Build history of the part. All positions in model axes, mm. Face numbers are marked on the shaded views. A direction names the side the tool comes from. Round coordinates to 2 decimals unless told otherwise and drop trailing zeros. Loops run counter-clockwise (first coordinate to the right, second up) from the corner with the lowest first, then second, coordinate; pieces in that order, holes last. Notation, with made-up numbers: (62.25, 37.25) - (104.25, 37.25) arc R17 cw to (104.25, 52.25) - close; hole circle Ø8 at (27, 53). An arc over 180 degrees is marked (long way). Put each result on its own line as item: value. Start each with the question number.
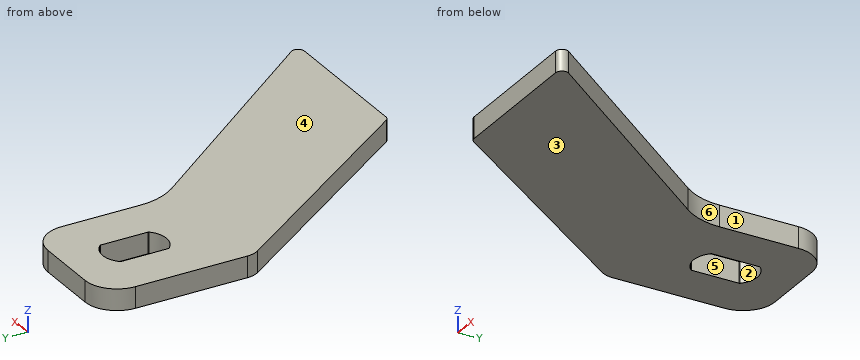
from build123d import *

# Parameters (mm, degrees)
EXTRUDE1_DEPTH = 10


with BuildPart() as part:
    # Sketch1 → Extrude1 (new body)
    with BuildSketch(Plane.XY):
        with BuildLine():
            Line((15, 32), (-15, 32))
            ThreePointArc((-15, 32), (-25.606601718, 27.606601718), (-30, 17))
            Line((-30, 17), (-30, -35.847012111))
            ThreePointArc((-30, -35.847012111), (-29.537169507, -38.854070106), (-28.191520443, -41.582776475))
            Line((-28.191520443, -41.582776475), (43.326244069, -143.720729309))
            ThreePointArc((43.326244069, -143.720729309), (44.398454362, -144.6610325), (45.783700202, -145))
            Line((45.783700202, -145), (111.775541918, -145))
            ThreePointArc((111.775541918, -145), (114.466160142, -143.326866071), (114.155601938, -140.173715713))
            Line((114.155601938, -140.173715713), (36.199399791, -38.579215104))
            ThreePointArc((36.199399791, -38.579215104), (31.592096115, -29.959556193), (30, -20.316372234))
            Line((30, -20.316372234), (30, 17))
            ThreePointArc((30, 17), (25.606601718, 27.606601718), (15, 32))
        make_face()
        with BuildLine():
            Line((8.25, -11.199832213), (8.25, 11.199832213))
            ThreePointArc((8.25, 11.199832213), (8.213806295, 11.386604055), (8.110465116, 11.546336037))
            ThreePointArc((8.110465116, 11.546336037), (0, 15), (-8.110465116, 11.546336037))
            ThreePointArc((-8.110465116, 11.546336037), (-8.213806295, 11.386604055), (-8.25, 11.199832213))
            Line((-8.25, 11.199832213), (-8.25, -11.199832213))
            ThreePointArc((-8.25, -11.199832213), (-8.213806295, -11.386604055), (-8.110465116, -11.546336037))
            ThreePointArc((-8.110465116, -11.546336037), (0, -15), (8.110465116, -11.546336037))
            ThreePointArc((8.110465116, -11.546336037), (8.213806295, -11.386604055), (8.25, -11.199832213))
        make_face(mode=Mode.SUBTRACT)
    extrude(amount=EXTRUDE1_DEPTH)


solid = part.part
Item 1: Slice it at A-A (z = 2.5). Give the cut face in (x, y).
Item 2: Slice it at B-B (x = 2.5). Give the cut face in (y, z), plus the area to 3 significant figures.
Item 3: Slice it at D-D (x = 59). Give the cut face in (y, z), plus the area to 3 significant figures.
Item 4: Which spindle directions (+Z, -Z, +X, -X, +Y, -Y) get a long thin tool onto all of the face, cutting with end or side? Do the marked faces 1, 2 and 3. Say none if no direction does.
Item 5: Two-plate mould, pull along Y, no slides. Class the marked faces 4, 5 and 6: pulls with the +Y half, pulls with the -Y half, needs draft (parallel to the pull), parting line crosses it, or undercut.
Item 6: Drill centre lines: probe 1 along X at (y, z) = (-5, 4.5); probe 2 along Y at (x, z) = (5, 7.5); probe 3 along Y at (x, z) = (33, 6.75). Where is each one in solid material? Low to high. Write a range as [from, to].
Item 7: Slice it at C-C (y = -73.5). Give the cut face in (x, z), plus the area to 3 significant figures.
Item 8: Drop flat-ended pins along their axis: pin 1 Ø5 at (x, y) = (92, -123) entering from -Z; pin 2 Ø4 at (y, z) = (-106.5, 8.5) entering from +X. Give the stop position or say it passes through.
Computed values:
1. outline: (-30, -35.85) arc R10 ccw to (-28.19, -41.58) - (43.33, -143.72) arc R3 ccw to (45.78, -145) - (111.78, -145) arc R3 ccw to (114.16, -140.17) - (36.2, -38.58) arc R30 cw to (30, -20.32) - (30, 17) arc R15 ccw to (15, 32) - (-15, 32) arc R15 ccw to (-30, 17) - close; hole (-8.25, -11.2) arc R0.5 ccw to (-8.11, -11.55) arc R11.25 ccw to (8.11, -11.55) arc R0.5 ccw to (8.25, -11.2) - (8.25, 11.2) arc R0.5 ccw to (8.11, 11.55) arc R11.25 ccw to (-8.11, 11.55) arc R0.5 ccw to (-8.25, 11.2) - close
2. outline: (-85.41, 0) - (-14.72, 0) - (-14.72, 10) - (-85.41, 10) - close; (14.72, 0) - (32, 0) - (32, 10) - (14.72, 10) - close
2. area: 880 mm^2
3. outline: (-145, 0) - (-68.29, 0) - (-68.29, 10) - (-145, 10) - close
3. area: 767 mm^2
4. face 1: +Z, -Z, +X, +Y
4. face 2: +Z, -Z
4. face 3: -Z, +X, -X, +Y, -Y
5. face 4: needs draft
5. face 5: undercut
5. face 6: pulls with the +Y half
6. probe 1: x = [-30, -8.25], [8.25, 30]
6. probe 2: y = [-88.99, -13.83], [13.83, 32]
6. probe 3: y = [-128.97, -33.39]
7. outline: (-5.84, 0) - (63, 0) - (63, 10) - (-5.84, 10) - close
7. area: 688 mm^2
8. pin 1: stops at z = 0
8. pin 2: stops at x = 89.85
